Model file for the job. Use its own axes, mm. A direction names the side the tool comes from. Give positions to 0.01 mm unless a question says otherwise; leave off trailing zeros. Write each loop counter-clockwise with the first axis right and the second up, starting at its lowest first coordinate (ties: lowest second). Pieces come first, ordered by that corner, then holes.
```python
from build123d import *

# Parameters (mm, degrees)
F0_W     = 50.8
F0_H     = 50.8
F1_DEPTH = 50.8
F2_W     = 46.3804
F2_H     = 46.7614
F3_DEPTH = 44.45
F4_W     = 47.35487
F4_H     = 46.960247
F5_DEPTH = 44.45


with BuildPart() as f1:
    # F0 (on Front) → F1 (new body)
    with BuildSketch(Plane.XZ):
        with Locations((25.4, -25.4)):
            Rectangle(F0_W, F0_H)
    extrude(amount=F1_DEPTH)

    # F2 (on Right) → F3 (cut)
    with BuildSketch(Plane.YZ):
        with Locations((-25.459287, -25.454011)):
            Rectangle(F2_W, F2_H)
    extrude(amount=-F3_DEPTH, mode=Mode.SUBTRACT)

    # F4 (on face) → F5 (cut)
    with BuildSketch(Plane.YZ.offset(50.8)):
        with Locations((-25.354586, -25.354588)):
            Rectangle(F4_W, F4_H)
    extrude(amount=-F5_DEPTH, mode=Mode.SUBTRACT)


solid = f1.part
```
1. Slice it at A-A, the plane x = 21.5. Write the cut outline in (y, z).
Calculated:
outline: (-50.8, -50.8) - (0, -50.8) - (0, 0) - (-50.8, 0) - close; hole (-49.03, -48.83) - (-1.68, -48.83) - (-1.68, -1.87) - (-49.03, -1.87) - close
2. Slice it at C-C, the plane z = -6.5. Write the cut outline in (x, y), and give its area (3 significant figures).
Calculated:
outline: (0, -50.8) - (50.8, -50.8) - (50.8, -49.03) - (6.35, -49.03) - (6.35, -1.68) - (50.8, -1.68) - (50.8, 0) - (0, 0) - close
area: 476 mm2
3. Pull direction Y, two halves, no side cores. Call faces 3 (the flat face through (50.8, -50, -27)), 4 (the flat face through (29, -26, -1.874)), 5 (the flat face through (25, -50.8, -25)), 6 (the flat face through (25, 0, -25)): +Y half, -Y half, draft (parallel to the pull), parting line (faces both ways), or undercut.
Calculated:
face 3: draft
face 4: undercut
face 5: -Y half
face 6: +Y half
4. Which spindle directions (+Z, -Z, +X, -X, +Y, -Y) get a long thin tool onto all of the face, cutting with end or side? Do faces 1 (the flat face through (29, -1.677, -26)), 2 (the flat face through (0, -25, -26)). Say none if no direction does.
Calculated:
face 1: +X
face 2: +Z, -Z, -X, +Y, -Y
5. Slice it at B-B, the plane y = -34. Write the cut outline in (x, z).
Calculated:
outline: (0, -50.8) - (50.8, -50.8) - (50.8, -48.83) - (6.35, -48.83) - (6.35, -1.87) - (50.8, -1.87) - (50.8, 0) - (0, 0) - close
6. Probe probe 1 along Z at (x, y) = (16.5, -36); probe 2 along Y at (x, z) = (28, -19.5); probe 3 along X at (y, z) = (-4, -31.5). List the from-to ranges inside material, lowest first.
Calculated:
probe 1: z = -50.8 to -48.83, -1.87 to 0
probe 2: y = -50.8 to -49.03, -1.68 to 0
probe 3: x = 0 to 6.35
7. Pin check, flat tip, straight feed: P1, Ø8, axis at y = -21.5, z = -41.5, coming from the +X side. Stop position of the tip, or through.
Calculated:
P1: stops at x = 6.35
